from build123d import *

# Parameters (mm, degrees)
F3_W     = 9.525
F3_H     = 25.1206
F4_DEPTH = 152.4


with BuildPart() as f1:
    # F0 (on Front) → F1 (revolve)
    with BuildSketch(Plane.XZ):
        Polygon((0, 0), (69.85, 0), (69.85, 25.4), (-21.05, 25.4), (-21.05, 38.1), (-97.25, 38.1), (-97.25, 0), align=None)
        Polygon((-264.35, 0), (-97.25, 0), (-97.25, 38.1), (-173.45, 38.1), (-173.45, 25.4), (-264.35, 25.4), align=None)
    revolve(axis=Axis((-97.25, 0, 0), (-1, 0, 0)))

    # F3 (on face) → F4 (cut, through all)
    with BuildSketch(Plane.YZ.offset(-21.05)):
        with Locations((0, 25.5397)):
            Rectangle(F3_W, F3_H)
        Polygon((-30.614318, -23.174446), (-8.85924, -10.614146), (-13.62174, -2.365254), (-35.376818, -14.925554), align=None)
        Polygon((35.376818, -14.925554), (13.62174, -2.365254), (8.85924, -10.614146), (30.614318, -23.174446), align=None)
    extrude(amount=-F4_DEPTH, mode=Mode.SUBTRACT)


solid = f1.part
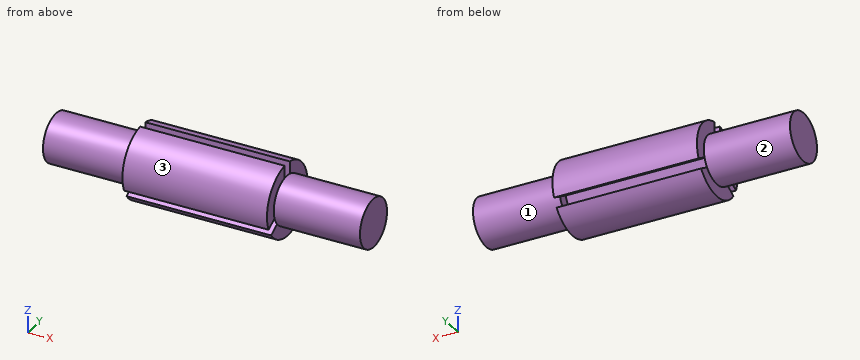
CAD build for the part. Positions are in the model's coordinates, mm. Face numbers are marked on the shaded views. A direction names the side the tool comes from. Give positions to 0.01 mm unless a question says otherwise; leave off trailing zeros. Order: outer loops, then holes, each group sorted by start corner. A loop starts at its lowest first (then second) coordinate and runs counter-clockwise, first axis right, second up. Notation, with made-up numbers: (-17.75, 36.25) - (7.25, 36.25) arc R11 cw to (7.25, 53.25) - close; hole circle Ø10 at (71.5, 43). An arc over 180 degrees is marked (long way). Write each question's results on one line, items separated by ' | '.
1. 3-axis set-ups, long thin cutter, end or side, ignore diameter. For the marked faces 1, 2 and 3: which of +Z, -Z, +X, -X, +Y, -Y reach the whole face in a straight line?
Calculated:
face 1: +X | face 2: -X | face 3: +X, -X, -Y
2. Saw through at B-B on x = -70. List the corners of the cut face in (y, z).
Calculated:
outline: (-35.12, -14.78) - (-13.62, -2.37) - (-8.86, -10.61) - (-30.36, -23.03) arc R38.1 ccw to (30.36, -23.03) - (8.86, -10.61) - (13.62, -2.37) - (35.12, -14.78) arc R38.1 ccw to (4.76, 37.8) - (4.76, 12.98) - (-4.76, 12.98) - (-4.76, 37.8) arc R38.1 ccw to start
3. Probe L1, parallel to Y at x = -46.5, z = -14.5; L2, parallel to X at y = -19.5, z = -13.5; L3, parallel to Y at x = 48, z = -0.5. List the from-to ranges inside material, lowest first. Write a range as from..to.
Calculated:
L1: y = -35.23..-34.64, -15.59..15.59, 34.64..35.23 | L2: x = -264.35..-173.45, -21.05..69.85 | L3: y = -25.4..25.4
4. Pin check, flat tips, straight feed: pin 1 (2 mm diameter, centred on y = -24, z = 16.5, fed in from -X); pin 2 (10 mm diameter, centred on x = 2.5, y = -6, fed in from -Z); pin 3 (10 mm diameter, centred on x = -90.5, z = -9, fed in from -Y). Stop position of each tip, or through.
Calculated:
pin 1: stops at x = -173.45 | pin 2: stops at z = -25.38 | pin 3: stops at y = -37.89
5. Saw through at A-A on y = 0. List the corners of the cut face in (x, z).
Calculated:
outline: (-264.35, -25.4) - (-173.45, -25.4) - (-173.45, -38.1) - (-21.05, -38.1) - (-21.05, -25.4) - (69.85, -25.4) - (69.85, 25.4) - (-21.05, 25.4) - (-21.05, 12.98) - (-173.45, 12.98) - (-173.45, 25.4) - (-264.35, 25.4) - close
6. Saw through at C-C on x = 48. List the corners of the cut face in (y, z).
Calculated:
outline: circle Ø50.8 at (0, 0)
